from build123d import *

# Parameters (mm, degrees)
F0_R           = 1.3992842893
F1_DEPTH       = 19.05
F2_R           = 5.08
F3_R           = 25.4
F4_R           = 1.3992842893
F5_DEPTH       = 19.05
F7_D           = 3.175
F7_CSINK_D     = 9.525
F7_CSINK_ANGLE = 90
F9_DEPTH       = 38.101
F11_DEPTH      = 19.05
F11_DEPTH_BACK = 19.05


with BuildPart() as f1:
    # F0 (on Front) → F1 (new body)
    with BuildSketch(Plane.XZ):
        with BuildLine():
            Line((150.8562757823, 76.2), (-166.6437242177, 76.2))
            Line((-166.6437242177, 76.2), (-166.6437242177, 0))
            Line((-166.6437242177, 0), (74.6562757823, 0))
            ThreePointArc((74.6562757823, 0), (106.2243540544, -10.8596763882), (130.1055285482, -34.187034615))
            Line((130.1055285482, -34.187034615), (150.8562757823, -66.1403832537))
            Line((150.8562757823, -66.1403832537), (150.8562757823, 76.2))
        make_face()
        with Locations((138.1562757823, -34.925)):
            Circle(F0_R, mode=Mode.SUBTRACT)
        with Locations((138.1562757823, -9.525)):
            Circle(F0_R, mode=Mode.SUBTRACT)
        with BuildLine():
            Line((78.4662757823, 33.3375), (-143.7837242177, 33.3375))
            ThreePointArc((-143.7837242177, 33.3375), (-148.5462242177, 38.1), (-143.7837242177, 42.8625))
            Line((-143.7837242177, 42.8625), (78.4662757823, 42.8625))
            ThreePointArc((78.4662757823, 42.8625), (83.2287757823, 38.1), (78.4662757823, 33.3375))
        make_face(mode=Mode.SUBTRACT)
        with Locations((138.1562757823, -34.925)):
            Circle(F0_R)
        with Locations((138.1562757823, -9.525)):
            Circle(F0_R)
    extrude(amount=F1_DEPTH)

    # F2
    f2_edges = [f1.edges().sort_by_distance(p)[0] for p in [
        (-166.643724, -9.525, 76.2),
        (-166.643724, -9.525, 0),
    ]]
    fillet(f2_edges, radius=F2_R)

    # F3
    f3_edges = [f1.edges().sort_by_distance(p)[0] for p in [
        (150.856276, -9.525, 76.2),
    ]]
    fillet(f3_edges, radius=F3_R)

    # F4 (on face) → F5 (join)
    with BuildSketch(Plane(origin=(0, 0, 0), x_dir=(-1, 0, 0), z_dir=(0, 1, 0))):
        with BuildLine():
            Line((-150.8562757823, 0), (-150.8562757823, -66.1403832537))
            Line((-150.8562757823, -66.1403832537), (-130.1055285482, -34.187034615))
            ThreePointArc((-130.1055285482, -34.187034615), (-106.2243540544, -10.8596763882), (-74.6562757823, 0))
            Line((-74.6562757823, 0), (-150.8562757823, 0))
        make_face()
        with Locations((-138.1562757823, -34.925)):
            Circle(F4_R, mode=Mode.SUBTRACT)
        with Locations((-138.1562757823, -9.525)):
            Circle(F4_R, mode=Mode.SUBTRACT)
        with Locations((-138.1562757823, -34.925)):
            Circle(F4_R)
        with Locations((-138.1562757823, -9.525)):
            Circle(F4_R)
    extrude(amount=F5_DEPTH)

    # F7 (through all)
    with Locations(Plane(origin=(0, 19.05, 0), x_dir=(-1, 0, 0), z_dir=(0, 1, 0))):
        with Locations((-138.1562757823, -34.925), (-138.1562757823, -9.525)):
            CounterSinkHole(F7_D / 2, F7_CSINK_D / 2, counter_sink_angle=F7_CSINK_ANGLE)

    # F8 (on face) → F9 (cut, through all)
    with BuildSketch(Plane.XZ.offset(19.05)):
        Polygon((150.8562757823, -66.1403832537), (150.8562757823, -2.6403832537), (149.3322757823, -2.6403832537), (149.3322757823, -63.7936290488), align=None)
    extrude(amount=-F9_DEPTH, mode=Mode.SUBTRACT)

    # F10 (on Front) → F11 (join, two sides)
    with BuildSketch(Plane.XZ) as f11_sk:
        with BuildLine():
            Line((150.8562757823, -63.7936290488), (150.8562757823, -2.6403832537))
            Line((150.8562757823, -2.6403832537), (149.3322757823, -2.6403832537))
            Line((149.3322757823, -2.6403832537), (149.3322757823, -63.7936290488))
            ThreePointArc((149.3322757823, -63.7936290488), (156.7895472638, -85.9779592892), (176.1329621077, -99.1532281041))
            ThreePointArc((176.1329621077, -99.1532281041), (177.0725432504, -98.6255205372), (176.5448356835, -97.6859393944))
            ThreePointArc((176.5448356835, -97.6859393944), (158.004098895, -85.0573940633), (150.8562757823, -63.7936290488))
        make_face()
    extrude(amount=F11_DEPTH)
    extrude(f11_sk.sketch, amount=-F11_DEPTH_BACK)


solid = f1.part
Can you work these out from the model? Positions are in its coordinate system, mm. A direction names the side the tool comes from. Give positions to 0.01 mm unless a question says otherwise; leave off trailing zeros. Loops run counter-clockwise (first coordinate to the right, second up) from the corner with the lowest first, then second, coordinate; pieces in that order, holes last. Notation, with made-up numbers: (-0.75, -7) -> (17.25, -7) arc R11 cw to (17.25, 11) -> close; hole circle Ø8 at (-35.5, 68.5). An arc over 180 degrees is marked (long way). Write item = value, one per line.
1) Will these pins go through, and if not, where does the flat tip stop? pin 1 (1.5 mm diameter, centred on y = 3, z = -20.5, fed in from +X); pin 2 (21 mm diameter, centred on x = 124.5, y = 13.5, fed in from +Z); pin 3 (6 mm diameter, centred on x = 78.5, z = 42, fed in from +Y); pin 4 (1.9 mm diameter, centred on x = 138.16, z = -34.92, fed in from -Y).
Check result:
pin_1 = 150.86
pin_2 = 0
pin_3 = 0
pin_4 = through
2) Suppose I cut it at B-B on z = 38.1. Write out the boundary of the cut face in (x, y).
Check result:
outline = (-166.64, -19.05) -> (-148.55, -19.05) -> (-148.55, 0) -> (-166.64, 0) -> close; (83.23, -19.05) -> (150.86, -19.05) -> (150.86, 0) -> (83.23, 0) -> close
3) Suppose I cut it at C-C on y = 7. Write out the boundary of the cut face in (x, z) (1 decimal).
Check result:
outline = (74.7, 0) arc R76.1 cw to (130.1, -34.2) -> (149.3, -63.8) arc R36.7 ccw to (176.1, -99.2) arc R0.8 ccw to (176.5, -97.7) arc R35.2 cw to (150.9, -63.8) -> (150.9, 0) -> close; hole circle Ø3.2 at (138.2, -34.9); hole circle Ø3.2 at (138.2, -9.5)
4) Thinking about a two-plate mould opening in Z: for faces 1 (the conical face through (139.093, 16.029, -8.056)), 2 (the cylindrical face through (143.218, -9.658, 68.957)), 3 (the flat face through (150.856, -5, -20)), which applies, released by +Z, released by -Z, zero draft, split by the parting line, or undercut?
Check result:
face_1 = undercut
face_2 = released by +Z
face_3 = zero draft
5) I need wall thicknesses on L1, parallel to Z at x = 38, y = -3; L2, parallel to X at y = 8, z = -66; L3, parallel to Y at x = 17, z = 21. Which ranges of each line are inside material? Lowest first, please. Write a range as from..to.
Check result:
L1 = 0..33.34, 42.86..76.2
L2 = 149.4..150.93
L3 = -19.05..0
6) For faces 4 (the flat face through (-45, -9, 0)), 5 (the flat face through (-31, -9, 33.338)), 6 (the flat face through (3, -19.05, 29)), 7 (the flat face through (112, 9, 0)), 8 (the cylindrical face through (158.198, -0.267, -85.311)), which set-ups out of +Z, -Z, +X, -X, +Y, -Y let a thin tool reach every point of the face, with its end or its side?
Check result:
face_4 = -Z, -X, +Y, -Y
face_5 = +Y, -Y
face_6 = +Z, -Z, +X, -X, -Y
face_7 = +Z, +X, -X, +Y
face_8 = +Z, +X, +Y, -Y
7) Suppose I cut it at A-A on x = -95.5. Write out the boundary of the cut face in (y, z).
Check result:
outline = (-19.05, 0) -> (0, 0) -> (0, 33.34) -> (-19.05, 33.34) -> close; (-19.05, 42.86) -> (0, 42.86) -> (0, 76.2) -> (-19.05, 76.2) -> close
8) Suppose I cut it at D-D on z = 19. Write out the boundary of the cut face in (x, y).
Check result:
outline = (-166.64, -19.05) -> (150.86, -19.05) -> (150.86, 0) -> (-166.64, 0) -> close
